The drawing under review shows one solid part. Ordinate dimensions are in mm from its lowest x, y, z. Round coordinates to 2 decimals unless told otherwise and drop trailing zeros. Order: outer loops, then holes, each group sorted by start corner. A loop starts at its lowest first (then second) coordinate and runs counter-clockwise, first axis right, second up. Notation, with made-up numbers: (4.25, -13) -> (37.25, -13) arc R19 ccw to (37.25, -1) -> close; hole circle Ø8 at (-29.5, -14). An arc over 180 degrees is marked (long way). Use a Markdown table: item, result. Add a question column.
1) Consider section A-A (z = 8.75). State the section outline as (x, y) points (1 decimal).
2) Draft analysis for pull direction X (two halves, no side actions). For the marked faces 1, 2 and 3, state which applies: pulls with the +X half, pulls with the -X half, needs draft (parallel to the pull), parting line crosses it, or undercut.
3) Clearance check with flat-ended pins moving along their axes: P1, Ø3, axis at y = 0.5, z = 6.5, coming from the +X side (1 decimal); P2, Ø2, axis at x = 1, y = 4.5, coming from the +Z side; P3, Ø2, axis at y = 3, z = 12, coming from the +X side. State where each tip first meets the part, or that it passes through.
4) Wall thickness on line 1 along X through (y, z) = (2.75, 11.75); line 2 along X through (y, z) = (3.5, 15.25) (1 decimal); line 3 along X through (y, z) = (1.5, 7.25): over which ranges is each line inside the solid? List them lowest first. Write a range as [from, to].
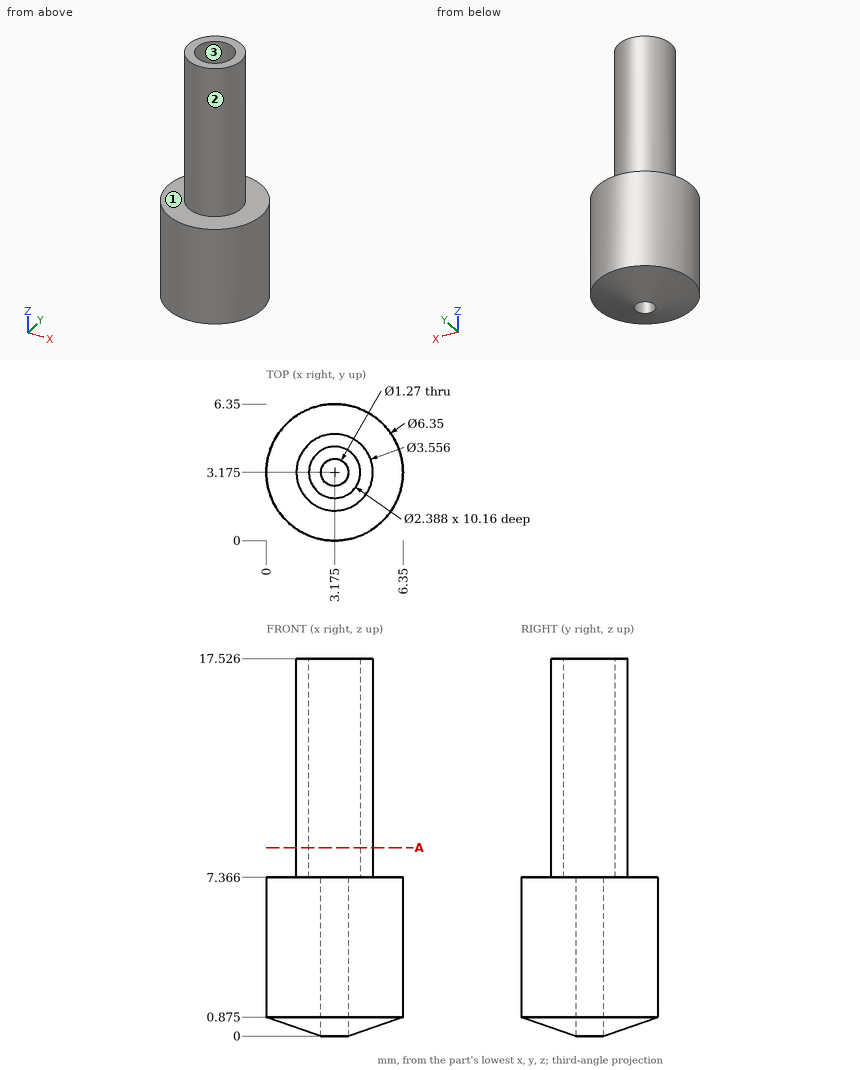
Results list:
| question | item | result |
|---|---|---|
| 1 | outline | circle Ø3.6 at (3.2, 3.2); hole circle Ø2.4 at (3.2, 3.2) |
| 2 | face 1 | needs draft |
| 2 | face 2 | parting line crosses it |
| 2 | face 3 | undercut |
| 3 | P1 | x = 6.1 |
| 3 | P2 | z = 17.53 |
| 3 | P3 | x = 4.95 |
| 4 | line 1 | [1.45, 2.06], [4.29, 4.9] |
| 4 | line 2 | [1.4, 2], [4.3, 4.9] |
| 4 | line 3 | [0.48, 5.87] |
